```python
from build123d import *

# Parameters (mm, degrees)
SKETCH001_W       = 69.1
SKETCH001_H       = 31.1
PAD_DEPTH         = 18.51
CYLINDER_R        = 11.5
CYLINDER_DEPTH    = 47
CYLINDER001_R     = 10.5
CYLINDER001_DEPTH = 45
BOX_W             = 67.1
BOX_H             = 29.1
BOX_DEPTH         = 17.51
SKETCH003_W       = 6
SKETCH003_H       = 4.5
SKETCH003_R       = 1
SKETCH003_H_2     = 6.5
PAD001_DEPTH      = 10.7
SKETCH004_W       = 8
SKETCH004_H       = 17.51
POCKET_DEPTH      = 5
SKETCH005_W       = 3
SKETCH005_H       = 13.55
PAD002_DEPTH      = 10.7
SKETCH006_W       = 19
SKETCH006_H       = 11.61
POCKET001_DEPTH   = 5
SKETCH007_W       = 22
SKETCH007_H       = 4.51
POCKET002_DEPTH   = 5


with BuildPart() as part:
    # Sketch001 → Pad (new body)
    with BuildSketch(Plane.XY):
        Rectangle(SKETCH001_W, SKETCH001_H)
    extrude(amount=PAD_DEPTH)

    # Cylinder → Cylinder (join)
    with BuildSketch(Plane(origin=(28.55, 0, 20.81), x_dir=(0, -1, 0), z_dir=(-1, 0, 0))):
        Circle(CYLINDER_R)
    extrude(amount=CYLINDER_DEPTH)

    # Cylinder001 → Cylinder001 (cut)
    with BuildSketch(Plane(origin=(27.55, 0, 20.81), x_dir=(0, 1, 0), z_dir=(-1, 0, 0))):
        Circle(CYLINDER001_R)
    extrude(amount=CYLINDER001_DEPTH, mode=Mode.SUBTRACT)

    # Box → Box (cut)
    with BuildSketch(Plane(origin=(-33.55, -14.55, 0), x_dir=(1, 0, 0), z_dir=(0, 0, 1))):
        with Locations((33.55, 14.55)):
            Rectangle(BOX_W, BOX_H)
    extrude(amount=BOX_DEPTH, mode=Mode.SUBTRACT)

    # Sketch003 (on Face15 of Box) → Pad001 (join)
    with BuildSketch(Plane(origin=(-33.55, -14.55, 17.51), x_dir=(1, 0, 0), z_dir=(0, 0, -1))):
        with Locations((64.1, -2.25)):
            Rectangle(SKETCH003_W, SKETCH003_H)
        with Locations((63.1, -2.5)):
            Circle(SKETCH003_R, mode=Mode.SUBTRACT)
        with Locations((64.1, -25.85)):
            Rectangle(SKETCH003_W, SKETCH003_H_2)
        with Locations((63.1, -24.6)):
            Circle(SKETCH003_R, mode=Mode.SUBTRACT)
    extrude(amount=PAD001_DEPTH)

    # Sketch004 (on Face2 of Pad001) → Pocket (cut)
    with BuildSketch(Plane(origin=(-33.55, 15.55, 0), x_dir=(-1, 0, 0), z_dir=(0, 1, 0))):
        with Locations((-15.5, 8.755)):
            Rectangle(SKETCH004_W, SKETCH004_H)
    extrude(amount=-POCKET_DEPTH, mode=Mode.SUBTRACT)

    # Sketch005 (on Face20 of Pocket) → Pad002 (join)
    with BuildSketch(Plane(origin=(-33.55, -14.55, 17.51), x_dir=(1, 0, 0), z_dir=(0, 0, -1))):
        with Locations((1.5, -13.55)):
            Rectangle(SKETCH005_W, SKETCH005_H)
    extrude(amount=PAD002_DEPTH)

    # Sketch006 (on Face3 of Pad002) → Pocket001 (cut)
    with BuildSketch(Plane(origin=(-33.55, -15.55, 0), x_dir=(1, 0, 0), z_dir=(0, -1, 0))):
        with Locations((15.5, 5.805)):
            Rectangle(SKETCH006_W, SKETCH006_H)
    extrude(amount=-POCKET001_DEPTH, mode=Mode.SUBTRACT)

    # Sketch007 (on Face1 of Pocket001) → Pocket002 (cut)
    with BuildSketch(Plane(origin=(-34.55, -14.55, 0), x_dir=(0, -1, 0), z_dir=(-1, 0, 0))):
        with Locations((-13.55, 2.255)):
            Rectangle(SKETCH007_W, SKETCH007_H)
    extrude(amount=-POCKET002_DEPTH, mode=Mode.SUBTRACT)


solid = part.part
```
Geometry: final body of the model. Coordinates: model frame, mm. A direction names the side the tool comes from. Coordinates: 2 decimals unless noted, no trailing zeros. Order: outer loops, then holes, each group sorted by start corner. A loop starts at its lowest first (then second) coordinate and runs counter-clockwise, first axis right, second up. Notation, with made-up numbers: (59, -5.5) -> (88, -5.5) arc R16 cw to (88, 22.5) -> close; hole circle Ø1 at (5, -21). An arc over 180 degrees is marked (long way). Use CSV: the item, a comma, the result in double quotes.
1) Line query: line 1 (X direction, y = 10.05, z = 12); line 2 (Y direction, x = 24, z = 13); line 3 (X direction, y = 3, z = 13). Output: solid intervals per line, ascending.
Findings:
line 1,"x = -34.55 to -33.55, 27.55 to 28.55, 30.55 to 34.55"
line 2,"y = -15.55 to -14.55, 14.55 to 15.55"
line 3,"x = -34.55 to -30.55, 33.55 to 34.55"
2) Access query for faces 4 (the cylindrical face through (5.365, -0.278, 31.306)), 5 (the flat face through (-32, -15, 0)), 6 (the flat face through (31, 8.05, 12)). Directions: +Z, -Z, +X, -X, +Y, -Y. A direction counts if a zero-diameter tool reaches every point of the face in a straight line with its end or side. Return the directions, or none.
Findings:
face 4,"none"
face 5,"-Z, +X, -X, +Y, -Y"
face 6,"-Z"
3) Pin query (flat end, axial travel): pin 1 Ø15 at (x, y) = (4, -6.5) entering from -Z; pin 2 Ø2 at (x, y) = (30, -12.5) entering from -Z; pin 3 Ø3 at (x, y) = (-7, 8) entering from -Z. Return the tip coordinate at first contact, or that it passes through.
Findings:
pin 1,"stops at z = 17.51"
pin 2,"stops at z = 6.81"
pin 3,"stops at z = 25.28"
4) Section B-B on x = -26. Output: boundary loops of the cut face in (y, z).
Findings:
outline,"(-15.55, 11.61) -> (-14.55, 11.61) -> (-14.55, 17.51) -> (14.55, 17.51) -> (14.55, 0) -> (15.55, 0) -> (15.55, 18.51) -> (-15.55, 18.51) -> close"
5) Section A-A on z = 9. Output: boundary loops of the cut face in (x, y) (3 decimals).
Findings:
outline,"(-34.55, -15.55) -> (-27.55, -15.55) -> (-27.55, -14.55) -> (-33.55, -14.55) -> (-33.55, -7.775) -> (-30.55, -7.775) -> (-30.55, 5.775) -> (-33.55, 5.775) -> (-33.55, 14.55) -> (-22.05, 14.55) -> (-22.05, 15.55) -> (-34.55, 15.55) -> close; (-14.05, 14.55) -> (27.55, 14.55) -> (27.55, 8.05) -> (33.55, 8.05) -> (33.55, -10.05) -> (27.55, -10.05) -> (27.55, -14.55) -> (-8.55, -14.55) -> (-8.55, -15.55) -> (34.55, -15.55) -> (34.55, 15.55) -> (-14.05, 15.55) -> close; hole circle Ø2 at (29.55, -12.05); hole circle Ø2 at (29.55, 10.05)"
6) Mould query, pull axis X, two halves, no side actions, for faces 1 (the flat face through (34.55, 0, 9)), 2 (the flat face through (-18.45, 0, 24)), 3 (the flat face through (-28, 14.55, 9)). Classes: +X half, -X half, draft (parallel to the pull), parting line (faces both ways), or undercut.
Findings:
face 1,"+X half"
face 2,"-X half"
face 3,"undercut"
7) Section C-C on z = 12.5. Output: boundary loops of the cut face in (x, y) (3 decimals), then the cut area to 3 significant figures.
Findings:
outline,"(-34.55, -15.55) -> (34.55, -15.55) -> (34.55, 15.55) -> (-14.05, 15.55) -> (-14.05, 14.55) -> (27.55, 14.55) -> (27.55, 8.05) -> (33.55, 8.05) -> (33.55, -10.05) -> (27.55, -10.05) -> (27.55, -14.55) -> (-33.55, -14.55) -> (-33.55, -7.775) -> (-30.55, -7.775) -> (-30.55, 5.775) -> (-33.55, 5.775) -> (-33.55, 14.55) -> (-22.05, 14.55) -> (-22.05, 15.55) -> (-34.55, 15.55) -> close; hole circle Ø2 at (29.55, -12.05); hole circle Ø2 at (29.55, 10.05)"
area,"289 mm^2"
8) Section D-D on y = 0. Output: boundary loops of the cut face in (x, z), then the cut area to 3 significant figures.
Findings:
outline,"(-34.55, 4.51) -> (-33.55, 4.51) -> (-33.55, 6.81) -> (-30.55, 6.81) -> (-30.55, 17.51) -> (-17.45, 17.51) -> (-17.45, 31.31) -> (27.55, 31.31) -> (27.55, 17.51) -> (33.55, 17.51) -> (33.55, 0) -> (34.55, 0) -> (34.55, 18.51) -> (28.55, 18.51) -> (28.55, 32.31) -> (-18.45, 32.31) -> (-18.45, 18.51) -> (-34.55, 18.51) -> close"
area,"159 mm^2"
